Input: part model. Units: mm. Frame: model coordinates. Face numbers are marked on the shaded views. A direction names the side the tool comes from. Round coordinates to 2 decimals unless told otherwise and drop trailing zeros. Write each loop counter-clockwise with the first axis right and the second up, starting at its lowest first coordinate (ties: lowest second). Pieces come first, ordered by that corner, then holes. Notation, with made-up numbers: (10.25, 22) - (16.25, 22) arc R34 cw to (16.25, 55) - close; hole circle Ø2 at (19, -9). An arc over 180 degrees is marked (long way). One line per item, written item: value. Start each with the question number.
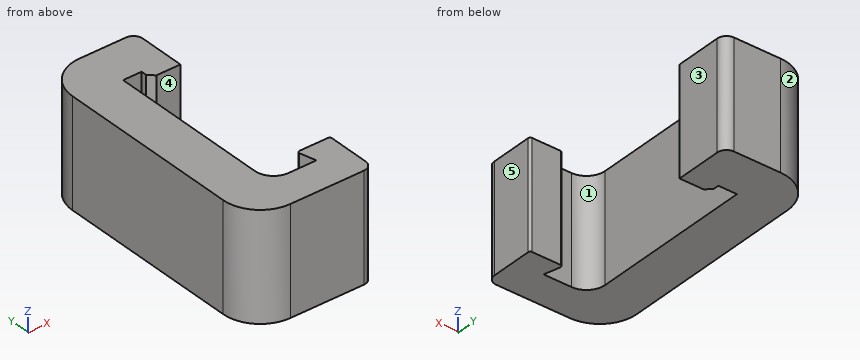
```python
from build123d import *

# Parameters (mm, degrees)
F1_DEPTH = 5.75
F2_R     = 0.5
F3_SIZE  = 0.3
F4_R     = 0.12


with BuildPart() as f1:
    # F0 (on Top) → F1 (new body)
    with BuildSketch(Plane.XY):
        with BuildLine():
            Line((-0.482554, 4.676151), (-0.482554, 4.076151))
            Line((-0.482554, 4.076151), (1.117446, 4.076151))
            Line((1.117446, 4.076151), (1.117446, 7.076151))
            Line((1.117446, 7.076151), (-1.882554, 7.076151))
            ThreePointArc((-1.882554, 7.076151), (-3.296768, 6.490364), (-3.882554, 5.076151))
            Line((-3.882554, 5.076151), (-3.882554, -4.923849))
            ThreePointArc((-3.882554, -4.923849), (-3.296768, -6.338063), (-1.882554, -6.923849))
            Line((-1.882554, -6.923849), (2.567446, -6.923849))
            Line((2.567446, -6.923849), (2.567446, -4.073849))
            Line((2.567446, -4.073849), (0.767446, -4.073849))
            Line((0.767446, -4.073849), (1.017446, -5.073849))
            Line((1.017446, -5.073849), (-0.482554, -5.073849))
            ThreePointArc((-0.482554, -5.073849), (-1.189661, -4.780956), (-1.482554, -4.073849))
            Line((-1.482554, -4.073849), (-1.482554, 4.676151))
            Line((-1.482554, 4.676151), (-0.482554, 4.676151))
        make_face()
    extrude(amount=F1_DEPTH)

    # F2
    f2_edges = [f1.edges().sort_by_distance(p)[0] for p in [
        (2.567446, -6.923849, 2.875),
        (1.117446, 7.076151, 2.875),
    ]]
    fillet(f2_edges, radius=F2_R)

    # F3
    f3_edges = [f1.edges().sort_by_distance(p)[0] for p in [
        (-0.482554, 4.076151, 2.875),
    ]]
    chamfer(f3_edges, length=F3_SIZE)

    # F4
    f4_edges = [f1.edges().sort_by_distance(p)[0] for p in [
        (0.767446, -4.073849, 2.875),
        (2.567446, -4.073849, 2.875),
    ]]
    fillet(f4_edges, radius=F4_R)


solid = f1.part
```
Q1. Contact query for flat-ended pins moving along their axis: pin 1 Ø1.5 at (y, z) = (-0.5, 3) entering from +X; pin 2 Ø2 at (y, z) = (5, 2) entering from +X; pin 3 Ø1.5 at (x, y) = (-2.5, -5) entering from -Z; pin 4 Ø0.8 at (x, z) = (2, 2.5) entering from +Y. Output: stop coordinate, or through.
Q2. Material intervals for probe 1 along Y at (x, z) = (0, 3.1); probe 2 along X at (y, z) = (1.75, 5.3); probe 3 along Y at (x, z) = (-1, 3.85), sorted ascending. Write a range as from..to.
Q3. Access query for the marked faces 4 and 5. Directions: +Z, -Z, +X, -X, +Y, -Y. A direction counts if a zero-diameter tool reaches every point of the face in a straight line with its end or side. Return the directions, or none.
Q4. Cut plane C-C, the plane y = -1.5. Output: boundary loops of the cut face in (x, z).
Q5. Pull-direction query (Y, two-part tool) for the marked faces 1, 2 and 3; classes: pulls with the +Y half, pulls with the -Y half, needs draft (parallel to the pull), parting line crosses it, or undercut.
Q6. Cut plane A-A, the plane z = 3.5. Output: boundary loops of the cut face in (x, y).
Q7. Cut plane B-B, the plane x = 1.75. Output: boundary loops of the cut face in (y, z), and give its area (3 significant figures).
A:
1. pin 1: stops at x = -1.48
1. pin 2: stops at x = 1.12
1. pin 3: stops at z = 0
1. pin 4: stops at y = -4.07
2. probe 1: y = -6.92..-5.07, 4.08..7.08
2. probe 2: x = -3.88..-1.48
2. probe 3: y = -6.92..-4.93, 4.68..7.08
3. face 4: +Z, -Z, +X
3. face 5: +Z, -Z, +X, +Y, -Y
4. outline: (-3.88, 0) - (-1.48, 0) - (-1.48, 5.75) - (-3.88, 5.75) - close
5. face 1: undercut
5. face 2: pulls with the +Y half
5. face 3: needs draft
6. outline: (-3.88, -4.92) arc R2 ccw to (-1.88, -6.92) - (2.07, -6.92) arc R0.5 ccw to (2.57, -6.42) - (2.57, -4.19) arc R0.12 ccw to (2.45, -4.07) - (0.92, -4.07) arc R0.12 ccw to (0.8, -4.22) - (1.02, -5.07) - (-0.48, -5.07) arc R1 cw to (-1.48, -4.07) - (-1.48, 4.68) - (-0.48, 4.68) - (-0.48, 4.38) - (-0.18, 4.08) - (1.12, 4.08) - (1.12, 6.58) arc R0.5 ccw to (0.62, 7.08) - (-1.88, 7.08) arc R2 ccw to (-3.88, 5.08) - close
7. outline: (-6.92, 0) - (-4.07, 0) - (-4.07, 5.75) - (-6.92, 5.75) - close
7. area: 16.4 mm²
